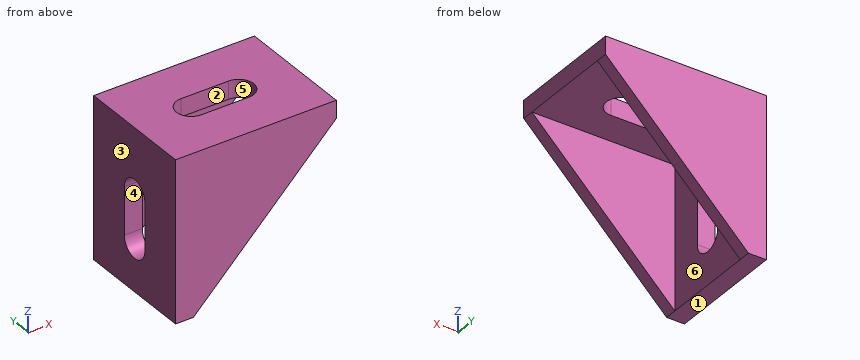
from build123d import *

# Parameters (mm, degrees)
SKETCH1_W           = 27
SKETCH1_H           = 20
BOSS_EXTRUDE1_DEPTH = 3
SKETCH2_W           = 3
SKETCH2_H           = 20
BOSS_EXTRUDE2_DEPTH = 24
BOSS_EXTRUDE3_DEPTH = 2
CUT_EXTRUDE1_DEPTH  = 3


with BuildPart() as part:
    # Sketch1 → Boss-Extrude1 (new body)
    with BuildSketch(Plane.XY):
        Rectangle(SKETCH1_W, SKETCH1_H)
        with BuildLine():
            Line((4, -2.5), (-4, -2.5))
            ThreePointArc((-4, -2.5), (-6.5, 0), (-4, 2.5))
            Line((-4, 2.5), (4, 2.5))
            ThreePointArc((4, 2.5), (6.5, 0), (4, -2.5))
        make_face(mode=Mode.SUBTRACT)
    extrude(amount=BOSS_EXTRUDE1_DEPTH)

    # Sketch2 → Boss-Extrude2 (add)
    with BuildSketch(Plane(origin=(0, 0, 0), x_dir=(-1, 0, 0), z_dir=(0, 0, -1))):
        with Locations((12, 0)):
            Rectangle(SKETCH2_W, SKETCH2_H)
    extrude(amount=BOSS_EXTRUDE2_DEPTH)

    # Sketch3 → Boss-Extrude3 (add)
    with BuildSketch(Plane.XZ.offset(10)):
        Polygon((-10.5, -24), (13.5, 0), (13.5, 3), (-13.5, 3), (-13.5, -24), align=None)
    boss_extrude3 = extrude(amount=-BOSS_EXTRUDE3_DEPTH)

    # Mirror1: Boss-Extrude3 across plane
    add(boss_extrude3.mirror(Plane.ZX))

    # Sketch4 → Cut-Extrude1 (cut)
    with BuildSketch(Plane(origin=(-10.5, 0, 0), x_dir=(0, 0, -1), z_dir=(1, 0, 0))):
        with BuildLine():
            Line((8, 2.5), (16, 2.5))
            ThreePointArc((16, 2.5), (18.5, 0), (16, -2.5))
            Line((16, -2.5), (8, -2.5))
            ThreePointArc((8, -2.5), (5.5, 0), (8, 2.5))
        make_face()
    extrude(amount=-CUT_EXTRUDE1_DEPTH, mode=Mode.SUBTRACT)


solid = part.part
Geometry: final body of the model. Coordinates: model frame, mm. Face numbers are marked on the shaded views. A direction names the side the tool comes from. Coordinates: 2 decimals unless noted, no trailing zeros. Order: outer loops, then holes, each group sorted by start corner. A loop starts at its lowest first (then second) coordinate and runs counter-clockwise, first axis right, second up. Notation, with made-up numbers: M 70.25,84.5 L 109.25,84.5 A32 cw 109.25,121.5 Z; hole C 65,73.5 d11. An arc over 180 degrees is marked long. One line per question, with ' | ' between items. Start each with the question number.
Item 1: Cut plane B-B, the plane y = 0.75. Return the cut outline in (x, z), then the cut area to 3 significant figures.
Item 2: Cut plane D-D, the plane z = -5. Return the cut outline in (x, y).
Item 3: Draft query along X for the marked faces 1, 2 and 3. Return one class per face: released by +X, released by -X, zero draft, split by the parting line, or undercut.
Item 4: Set-up query: the marked faces 4, 5 and 6. Return all of +Z, -Z, +X, -X, +Y, -Y with unobstructed straight access to the full face (end or side cutting, diameter ignored); none if empty.
Item 5: Cut plane A-A, the plane z = -8.5. Return the cut outline in (x, y).
Item 6: Pin query (flat end, axial travel): pin 1 Ø7 at (x, z) = (4.5, -11) entering from +Y; pin 2 Ø5 at (x, y) = (7, 0.5) entering from -Z. Return the tip coordinate at first contact, or that it passes through.
Item 7: Cut plane C-C, the plane x = 7. Return the cut outline in (y, z).
Item 8: Ray query, probe 1 along Y at (x, z) = (-8.75, -21.25); probe 2 along Z at (x, y) = (-7, 4.75); probe 3 along X at (y, z) = (3, -7.5). Return the intervals inside material, ascending. Write a range as [from, to].
A:
1) outline: M -13.5,-24 L -10.5,-24 L -10.5,-18.38 L -13.5,-18.38 Z; M -13.5,-5.62 L -10.5,-5.62 L -10.5,0 L -6.38,0 L -6.38,3 L -13.5,3 Z; M 6.38,0 L 13.5,0 L 13.5,3 L 6.38,3 Z | area: 76.4 mm2
2) outline: M -13.5,-10 L 8.5,-10 L 8.5,-8 L -10.5,-8 L -10.5,8 L 8.5,8 L 8.5,10 L -13.5,10 Z
3) face 1: zero draft | face 2: undercut | face 3: released by -X
4) face 4: +X, -X | face 5: +Z, -Z | face 6: -Z, +X
5) outline: M -13.5,-10 L 5,-10 L 5,-8 L -10.5,-8 L -10.5,-2.5 L -13.5,-2.5 Z; M -13.5,2.5 L -10.5,2.5 L -10.5,8 L 5,8 L 5,10 L -13.5,10 Z
6) pin 1: stops at y = 10 | pin 2: stops at z = 0
7) outline: M -10,-6.5 L -8,-6.5 L -8,0 L 8,0 L 8,-6.5 L 10,-6.5 L 10,3 L -10,3 Z
8) probe 1: y = [-10, -8], [8, 10] | probe 2: z = [0, 3] | probe 3: x = [-13.5, -10.5]
